Drawing for the job (mm, zero at the part's lowest x, y, z). A direction names the side the tool comes from. Give positions to 0.01 mm unless a question says otherwise; leave off trailing zeros. Write each loop counter-clockwise with the first axis right and the second up, starting at its lowest first coordinate (ties: lowest second). Pieces come first, ordered by that corner, then holes. Notation, with made-up numbers: M 43,79 L 67,79 A32 ccw 67,105 Z; hole C 68.25,35 d1. An arc over 180 degrees is marked long. Answer as a JSON object with one key per item and string values. Group by question number.
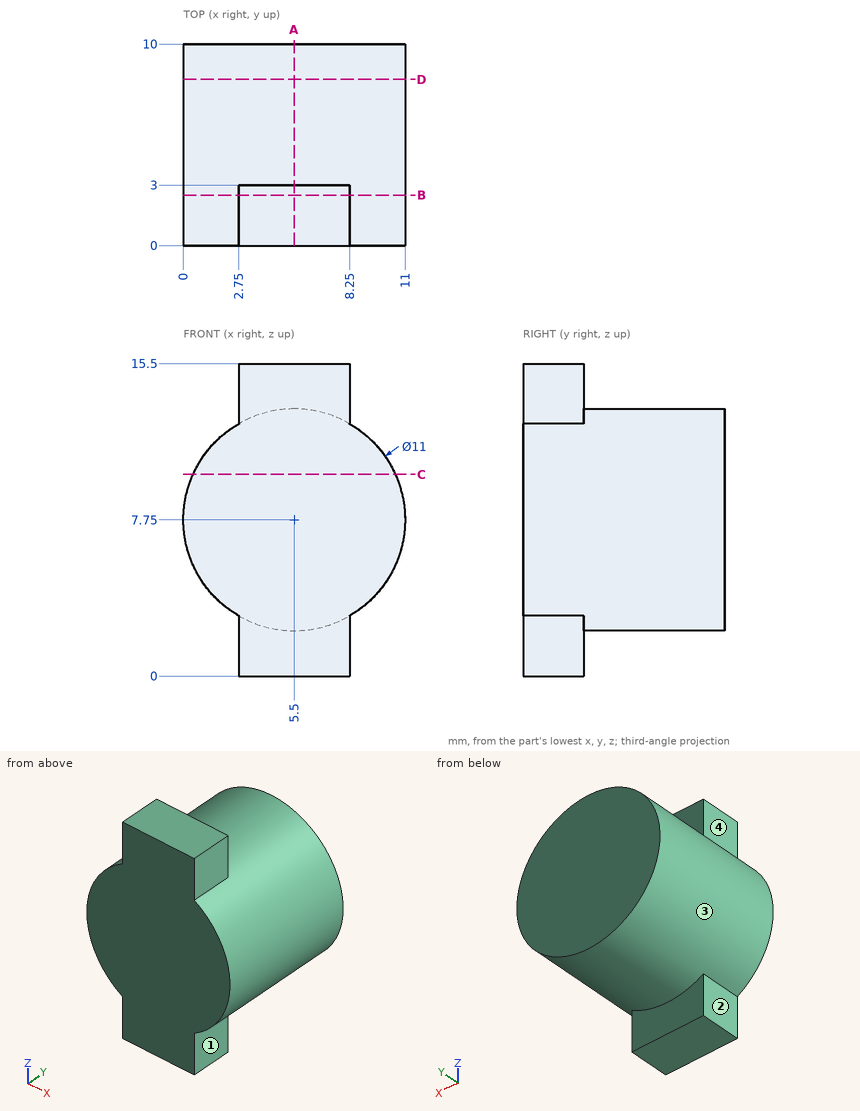
Q1. 3-axis set-ups, long thin cutter, end or side, ignore diameter. For the marked faces 1, 2, 3 and 4: which of +Z, -Z, +X, -X, +Y, -Y reach the whole face in a straight line?
Q2. Slice it at D-D, the plane y = 8.25. Write the cut outline in (x, z).
Q3. Slice it at C-C, the plane z = 10. Write the cut outline in (x, y), then the cut area to 3 significant figures.
Q4. Wall check: L1, parallel to Z at x = 8.25, y = 4.25; L2, parallel to Y at x = 3.25, z = 13.5; L3, parallel to Z at x = 1.5, y = 9.25. Give the ranges that are in metal, low to high.
Q5. Slice it at A-A, the plane x = 5.5. Write the cut outline in (y, z), then the cut area to 4 significant figures.
Q6. Slice it at B-B, the plane y = 2.5. Write the cut outline in (x, z).
Q7. Drop flat-ended pins along their axis: P1, Ø2.5, axis at y = 1.5, z = 13.5, coming from the -X side; P2, Ø1.5, axis at x = 3, y = 4.5, coming from the +Z side; P3, Ø3.5, axis at y = 2, z = 2, coming from the -X side. Give the stop position or say it passes through.
Solved:
{
 "1": {"face 1": "-Z, +X, +Y, -Y", "face 2": "-Z, -X, +Y, -Y", "face 3": "+Y", "face 4": "+Z, -X, +Y, -Y"},
 "2": {"outline": "C 5.5,7.75 d11"},
 "3": {"outline": "M 0.48,0 L 10.52,0 L 10.52,10 L 0.48,10 Z", "area": "100 mm²"},
 "4": {"L1": "z = 2.99 to 12.51", "L2": "y = 0 to 3", "L3": "z = 3.98 to 11.52"},
 "5": {"outline": "M 0,0 L 3,0 L 3,2.25 L 10,2.25 L 10,13.25 L 3,13.25 L 3,15.5 L 0,15.5 Z", "area": "123.5 mm²"},
 "6": {"outline": "M 2.75,0 L 8.25,0 L 8.25,2.99 A5.5 ccw 8.25,12.51 L 8.25,15.5 L 2.75,15.5 L 2.75,12.51 A5.5 ccw 2.75,2.99 Z"},
 "7": {"P1": "stops at x = 2.34", "P2": "stops at z = 12.96", "P3": "stops at x = 1.73"}
}
